Source: CAD feature listing. Evaluate the final solid. Frame: model axes, mm. Face numbers are marked on the shaded views. A direction names the side the tool comes from. Give positions to 0.01 mm unless a question says otherwise; leave off trailing zeros. Order: outer loops, then holes, each group sorted by start corner. A loop starts at its lowest first (then second) coordinate and runs counter-clockwise, first axis right, second up. Notation, with made-up numbers: M 3.5,48 L 56.5,48 A25 cw 56.5,66 Z; hole C 75,48.25 d2. An arc over 180 degrees is marked long. Use CSV: the item, a comma, the result in double quotes. Start each with the question number.
Item 1: Access query for the marked faces 1 and 2. Directions: +Z, -Z, +X, -X, +Y, -Y. A direction counts if a zero-diameter tool reaches every point of the face in a straight line with its end or side. Return the directions, or none.
Item 2: Ray query, probe 1 along X at (y, z) = (1.1, -21); probe 2 along Z at (x, y) = (-13.5, 1.8); probe 3 along Y at (x, z) = (-10.25, -23.5). Return the intervals inside material, ascending. Write a range as from..to.
Item 3: Section query B-B on z = -21. Return loops of the section in (x, y), and give its area (3 significant figures).
Item 4: First-contact query: pin 1 (6 mm diameter, centred on x = -15, z = -21, fed in from -Y); pin 2 (1.5 mm diameter, centred on x = -9.5, z = -16.5, fed in from -Y); pin 3 (1.5 mm diameter, centred on x = -11.5, z = -20.5, fed in from -Y). Flat tips, straight axial feed; report the tip coordinate or a pass-through.
Item 5: Section query C-C on y = 1.35. Return loops of the section in (x, z), and give its area (3 significant figures).
Item 6: Section query A-A on x = -13. Return loops of the section in (y, z).
Item 7: Section query D-D on x = -8.5. Return loops of the section in (y, z).
Item 8: Pull-direction query (Z, two-part tool) for the marked faces 3, 4 and 5; classes: +Z half, -Z half, draft (parallel to the pull), parting line (faces both ways), or undercut.
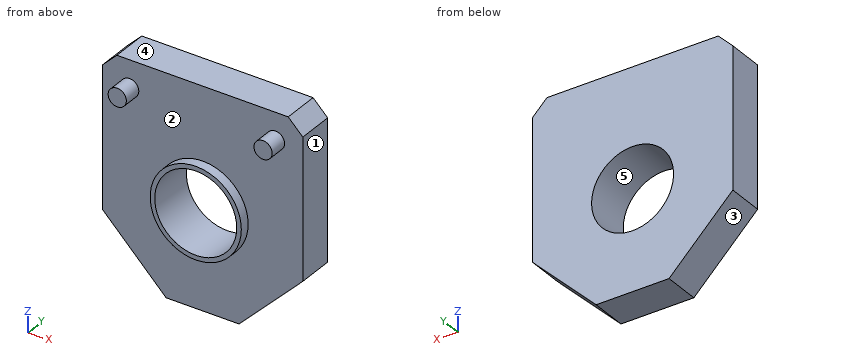
from build123d import *

# Parameters (mm, degrees)
SKETCH1_R           = 2.25
BOSS_EXTRUDE1_DEPTH = 2
SKETCH2_R           = 2.5
SKETCH2_R_2         = 2.25
BOSS_EXTRUDE2_DEPTH = 0.55
SKETCH3_R           = 0.5
BOSS_EXTRUDE3_DEPTH = 1


with BuildPart() as part:
    # Sketch1 → Boss-Extrude1 (new body)
    with BuildSketch(Plane(origin=(0, 0, 0), x_dir=(1, 0, 0), z_dir=(0, 1, 0))):
        Polygon((-17.906062461, 15.839978331), (-17.906062461, 23.539978331), (-14.406062461, 27.039978331), (-10.406062461, 27.039978331), (-6.906062461, 23.539978331), (-6.906062461, 15.839978331), (-7.706062461, 15.039978331), (-17.106062461, 15.039978331), align=None)
        with Locations((-12.406062461, 21.539978331)):
            Circle(SKETCH1_R, mode=Mode.SUBTRACT)
    extrude(amount=BOSS_EXTRUDE1_DEPTH)

    # Sketch2 → Boss-Extrude2 (add)
    with BuildSketch(Plane.XZ):
        with Locations((-12.406062461, -21.539978331)):
            Circle(SKETCH2_R)
        with Locations((-12.406062461, -21.539978331)):
            Circle(SKETCH2_R_2, mode=Mode.SUBTRACT)
    extrude(amount=BOSS_EXTRUDE2_DEPTH)

    # Sketch3 → Boss-Extrude3 (add)
    with BuildSketch(Plane.XZ):
        with Locations((-16.406062461, -16.539978331)):
            Circle(SKETCH3_R)
        with Locations((-8.406062461, -16.539978331)):
            Circle(SKETCH3_R)
    extrude(amount=BOSS_EXTRUDE3_DEPTH)


solid = part.part
Verdict:
1,face 1,"+Z, -Z, +X, +Y, -Y"
1,face 2,"-Y"
2,probe 1,"-17.91..-14.59, -10.22..-6.91"
2,probe 2,"-27.04..-23.51, -19.57..-15.04"
2,probe 3,"0..2"
3,outline,"M -17.91,0 L -14.85,0 L -14.85,-0.55 L -14.59,-0.55 L -14.59,2 L -17.91,2 Z; M -10.22,-0.55 L -9.97,-0.55 L -9.97,0 L -6.91,0 L -6.91,2 L -10.22,2 Z"
3,area,"13.5 mm2"
4,pin 1,"y = -0.55"
4,pin 2,"y = -1"
4,pin 3,"through"
5,outline,"M -17.91,-23.54 L -14.41,-27.04 L -10.41,-27.04 L -6.91,-23.54 L -6.91,-15.84 L -7.71,-15.04 L -17.11,-15.04 L -17.91,-15.84 Z; hole C -12.41,-21.54 d4.5"
5,area,"103 mm2"
6,outline,"M -0.55,-23.97 L 0,-23.97 L 0,-27.04 L 2,-27.04 L 2,-23.71 L -0.55,-23.71 Z; M -0.55,-19.37 L 2,-19.37 L 2,-15.04 L 0,-15.04 L 0,-19.11 L -0.55,-19.11 Z"
7,outline,"M -1,-17.03 L 0,-17.03 L 0,-25.13 L 2,-25.13 L 2,-15.04 L 0,-15.04 L 0,-16.05 L -1,-16.05 Z"
8,face 3,"-Z half"
8,face 4,"+Z half"
8,face 5,"undercut"
